Answer from the drawing. Dimensions are ordinates in mm from the lowest x, y and z of the part. A direction names the side the tool comes from. Round coordinates to 2 decimals unless told otherwise and drop trailing zeros. Write each loop counter-clockwise with the first axis right and the second up, starting at its lowest first coordinate (ties: lowest second). Pieces come first, ordered by that corner, then holes. Notation, with made-up numbers: M -17,-25 L 41,-25 A16 ccw 41,-11 Z; hole C 71.5,59 d6. An arc over 180 degrees is marked long. One line per item, written item: value. Start each with the question number.
(1) Given P1, Ø1.6, axis at y = 2, z = 4, coming from the +X side; P2, Ø1.6, axis at x = 13.5, y = 1.5, coming from the -Z side; P3, Ø1, axis at x = 9, y = 2, coming from the +Z side, each flat-ended and moving along its own axis, determine where each tip first touches the part or whether it passes through.
(2) Section D-D (z = 20) is taken. Determine the outline of the cut face in (x, y) (1 decimal), plus the area to 3 significant figures.
(3) For a pull along X with two mould halves and no side action, classify the marked faces 3, 4 and 5 as released by +X, released by -X, zero draft, split by the parting line, or undercut.
(4) Section B-B (y = 1.5) is taken. State how many separate pieces and enclosed holes the cut face has, plus the area to 3 significant figures.
(5) Section C-C (x = 17) is taken. Determine the outline of the cut face in (y, z) (3 decimals), plus the area to 3 significant figures.
(6) Section A-A (x = 30) is taken. Determine the outline of the cut face in (y, z) (1 decimal).
(7) Consider probe 1 along X at (y, z) = (1.7, 6.25); probe 2 along X at (y, z) = (1.9, 1.5) (1 decimal); probe 3 along Z at (x, y) = (18, 0.4). Determine where each line is inside the solid, lowest interval first.
(8) For the marked faces 1 and 2, determine the directions among +Z, -Z, +X, -X, +Y, -Y from which every point of the face is accessible in a straight line to the end or side of a thin tool.
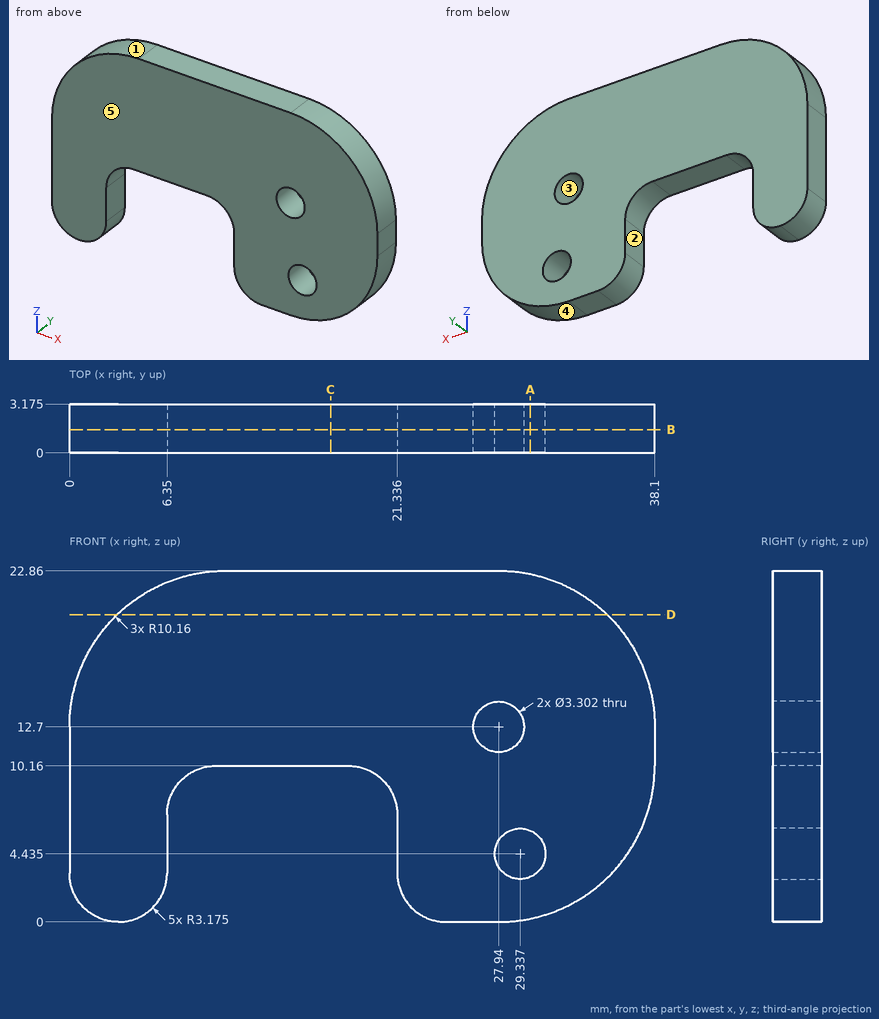
Recorded:
1. P1: stops at x = 36.57
1. P2: stops at z = 10.16
1. P3: stops at z = 22.84
2. outline: M 3.1,0 L 35,0 L 35,3.2 L 3.1,3.2 Z
2. area: 101 mm2
3. face 3: undercut
3. face 4: released by +X
3. face 5: zero draft
4. separate pieces: 1
4. enclosed holes: 2
4. area: 633 mm2
5. outline: M 0,10.16 L 3.175,10.16 L 3.175,22.86 L 0,22.86 Z
5. area: 40.3 mm2
6. outline: M 0,0.2 L 3.2,0.2 L 3.2,2.9 L 0,2.9 Z; M 0,5.9 L 3.2,5.9 L 3.2,22.6 L 0,22.6 Z
7. probe 1: x = 0 to 6.35, 21.34 to 37.32
7. probe 2: x = 0.5 to 5.9, 21.8 to 33.3
7. probe 3: z = 10.16 to 22.86
8. face 1: +Z, -X, +Y, -Y
8. face 2: -Z, +Y, -Y
